Here's how the part is built. I have some questions about the finished solid (model axes, mm). Coordinates: 2 decimals unless noted, no trailing zeros. Write each loop counter-clockwise with the first axis right and the second up, starting at its lowest first coordinate (ties: lowest second). Pieces come first, ordered by that corner, then holes. Notation, with made-up numbers: M 33.5,6 L 59.5,6 A24 ccw 59.5,32 Z; hole C 35,24 d2. An arc over 180 degrees is marked long. Use one line per item in the form item = value. Start each with the question number.
1. I want a section at A-A, the plane y = -3.5. List the corners of the cut face in (x, z) for me.
2. I want a section at B-B, the plane y = 3. List the corners of the cut face in (x, z) for me, plus the area to 3 significant figures.
3. Please list where these lines run through material, in increasing order: line 1 along X through (y, z) = (2, 3.75); line 2 along X through (y, z) = (-1.75, 0.9); line 3 along Y through (x, z) = (0.75, 0.8). Write a range as [from, to].
4. Thinking about a two-plate mould opening in X: for faces 1 (the face through (2, -2, 0)), 2 (the face through (-0.6, 4.415, 1.972)), which applies, released by +X, released by -X, zero draft, split by the parting line, or undercut?
5. I'm going to push flat-ended pins straight in: pin 1 Ø2 at (x, z) = (1.5, 3) entering from +Y; pin 2 Ø1 at (y, z) = (-3.5, 1.5) entering from -X. Where does each tip first touch, or does it pass through?
from build123d import *

# Parameters (mm, degrees)
F0_R     = 4.49904
F1_DEPTH = 4


with BuildPart() as f1:
    # F0 (on Top) → F1 (new body)
    with BuildSketch(Plane.XY):
        with Locations((-0.014088, -0.045997)):
            Circle(F0_R)
        with BuildLine():
            ThreePointArc((1.873632, 0.614697), (1.909564, 0.501329), (1.938694, 0.386026))
            Line((1.938694, 0.386026), (2.203247, 0.410541))
            ThreePointArc((2.203247, 0.410541), (2.386026, 0.353941), (2.475248, 0.184674))
            ThreePointArc((2.475248, 0.184674), (2.418648, 0.001895), (2.249381, -0.087326))
            Line((2.249381, -0.087326), (1.984828, -0.111841))
            ThreePointArc((1.984828, -0.111841), (1.977381, -0.230533), (1.962892, -0.348573))
            Line((1.962892, -0.348573), (2.218436, -0.421282))
            ThreePointArc((2.218436, -0.421282), (2.368426, -0.540087), (2.390476, -0.730154))
            ThreePointArc((2.390476, -0.730154), (2.271671, -0.880144), (2.081604, -0.902195))
            Line((2.081604, -0.902195), (1.82606, -0.829486))
            ThreePointArc((1.82606, -0.829486), (1.776239, -0.937473), (1.720087, -1.042308))
            Line((1.720087, -1.042308), (1.93211, -1.20242))
            ThreePointArc((1.93211, -1.20242), (2.028581, -1.36415), (1.984828, -1.547313))
            ThreePointArc((1.984828, -1.547313), (1.819226, -1.649054), (1.630792, -1.601429))
            Line((1.630792, -1.601429), (1.41877, -1.441317))
            ThreePointArc((1.41877, -1.441317), (1.333304, -1.524015), (1.243073, -1.601486))
            Line((1.243073, -1.601486), (1.382939, -1.827377))
            ThreePointArc((1.382939, -1.827377), (1.413744, -2.016223), (1.301993, -2.17154))
            ThreePointArc((1.301993, -2.17154), (1.113147, -2.202345), (0.95783, -2.090593))
            Line((0.95783, -2.090593), (0.817964, -1.864702))
            ThreePointArc((0.817964, -1.864702), (0.708396, -1.910941), (0.596272, -1.950586))
            Line((0.596272, -1.950586), (0.645092, -2.211749))
            ThreePointArc((0.645092, -2.211749), (0.605598, -2.39897), (0.445286, -2.503429))
            ThreePointArc((0.445286, -2.503429), (0.258065, -2.463936), (0.153605, -2.303624))
            Line((0.153605, -2.303624), (0.104786, -2.042461))
            ThreePointArc((0.104786, -2.042461), (-0.014088, -2.045997), (-0.132961, -2.042461))
            Line((-0.132961, -2.042461), (-0.181781, -2.303624))
            ThreePointArc((-0.181781, -2.303624), (-0.28624, -2.463936), (-0.473461, -2.503429))
            ThreePointArc((-0.473461, -2.503429), (-0.633773, -2.39897), (-0.673267, -2.211749))
            Line((-0.673267, -2.211749), (-0.624448, -1.950586))
            ThreePointArc((-0.624448, -1.950586), (-0.736571, -1.910941), (-0.84614, -1.864702))
            Line((-0.84614, -1.864702), (-0.986006, -2.090593))
            ThreePointArc((-0.986006, -2.090593), (-1.141322, -2.202345), (-1.330168, -2.17154))
            ThreePointArc((-1.330168, -2.17154), (-1.44192, -2.016223), (-1.411114, -1.827377))
            Line((-1.411114, -1.827377), (-1.271248, -1.601486))
            ThreePointArc((-1.271248, -1.601486), (-1.361479, -1.524015), (-1.446945, -1.441317))
            Line((-1.446945, -1.441317), (-1.658968, -1.601429))
            ThreePointArc((-1.658968, -1.601429), (-1.847401, -1.649054), (-2.013004, -1.547313))
            ThreePointArc((-2.013004, -1.547313), (-2.056756, -1.36415), (-1.960285, -1.20242))
            Line((-1.960285, -1.20242), (-1.748263, -1.042308))
            ThreePointArc((-1.748263, -1.042308), (-1.804414, -0.937473), (-1.854236, -0.829486))
            Line((-1.854236, -0.829486), (-2.10978, -0.902195))
            ThreePointArc((-2.10978, -0.902195), (-2.299846, -0.880144), (-2.418652, -0.730154))
            ThreePointArc((-2.418652, -0.730154), (-2.396601, -0.540087), (-2.246611, -0.421282))
            Line((-2.246611, -0.421282), (-1.991067, -0.348573))
            ThreePointArc((-1.991067, -0.348573), (-2.005556, -0.230533), (-2.013004, -0.111841))
            Line((-2.013004, -0.111841), (-2.277557, -0.087326))
            ThreePointArc((-2.277557, -0.087326), (-2.446823, 0.001895), (-2.503423, 0.184674))
            ThreePointArc((-2.503423, 0.184674), (-2.414201, 0.353941), (-2.231422, 0.410541))
            Line((-2.231422, 0.410541), (-1.966869, 0.386026))
            ThreePointArc((-1.966869, 0.386026), (-1.937739, 0.501329), (-1.901807, 0.614697))
            Line((-1.901807, 0.614697), (-2.13964, 0.733124))
            ThreePointArc((-2.13964, 0.733124), (-2.263982, 0.878126), (-2.246611, 1.068349))
            ThreePointArc((-2.246611, 1.068349), (-2.105122, 1.193314), (-1.91677, 1.180705))
            Line((-1.91677, 1.180705), (-1.678938, 1.062279))
            ThreePointArc((-1.678938, 1.062279), (-1.610122, 1.159273), (-1.535663, 1.252005))
            Line((-1.535663, 1.252005), (-1.714655, 1.448349))
            ThreePointArc((-1.714655, 1.448349), (-1.779903, 1.616773), (-1.714655, 1.785197))
            ThreePointArc((-1.714655, 1.785197), (-1.529903, 1.866773), (-1.345151, 1.785197))
            Line((-1.345151, 1.785197), (-1.166159, 1.588853))
            ThreePointArc((-1.166159, 1.588853), (-1.066952, 1.654438), (-0.964022, 1.71401))
            Line((-0.964022, 1.71401), (-1.059999, 1.961755))
            ThreePointArc((-1.059999, 1.961755), (-1.05558, 2.153046), (-0.917192, 2.285184))
            ThreePointArc((-0.917192, 2.285184), (-0.725901, 2.280764), (-0.593763, 2.142376))
            Line((-0.593763, 2.142376), (-0.497786, 1.894631))
            ThreePointArc((-0.497786, 1.894631), (-0.381587, 1.919949), (-0.264088, 1.938317))
            Line((-0.264088, 1.938317), (-0.264088, 2.204003))
            ThreePointArc((-0.264088, 2.204003), (-0.190864, 2.38078), (-0.014088, 2.454003))
            ThreePointArc((-0.014088, 2.454003), (0.162689, 2.38078), (0.235912, 2.204003))
            Line((0.235912, 2.204003), (0.235912, 1.938317))
            ThreePointArc((0.235912, 1.938317), (0.353411, 1.919949), (0.469611, 1.894631))
            Line((0.469611, 1.894631), (0.565588, 2.142376))
            ThreePointArc((0.565588, 2.142376), (0.697726, 2.280764), (0.889016, 2.285184))
            ThreePointArc((0.889016, 2.285184), (1.027405, 2.153046), (1.031824, 1.961755))
            Line((1.031824, 1.961755), (0.935847, 1.71401))
            ThreePointArc((0.935847, 1.71401), (1.038777, 1.654438), (1.137983, 1.588853))
            Line((1.137983, 1.588853), (1.316975, 1.785197))
            ThreePointArc((1.316975, 1.785197), (1.501728, 1.866773), (1.68648, 1.785197))
            ThreePointArc((1.68648, 1.785197), (1.751728, 1.616773), (1.68648, 1.448349))
            Line((1.68648, 1.448349), (1.507488, 1.252005))
            ThreePointArc((1.507488, 1.252005), (1.581947, 1.159273), (1.650762, 1.062279))
            Line((1.650762, 1.062279), (1.888595, 1.180705))
            ThreePointArc((1.888595, 1.180705), (2.076947, 1.193314), (2.218436, 1.068349))
            ThreePointArc((2.218436, 1.068349), (2.235807, 0.878126), (2.111464, 0.733124))
            Line((2.111464, 0.733124), (1.873632, 0.614697))
        make_face(mode=Mode.SUBTRACT)
    extrude(amount=F1_DEPTH)


solid = f1.part
Answer list:
q1.outline = M -2.9,0 L 2.87,0 L 2.87,4 L -2.9,4 Z
q2.outline = M -3.33,0 L 3.3,0 L 3.3,4 L -3.33,4 Z
q2.area = 26.5 mm²
q3.line_1 = [-4.02, -1.07], [-0.54, -0.26], [0.24, 0.51], [1.04, 3.99]
q3.line_2 = [-4.18, -1.36], [1.34, 4.15]
q3.line_3 = [-4.48, -1.89], [2.3, 4.39]
q4.face_1 = zero draft
q4.face_2 = split by the parting line
q5.pin_1 = 4.42
q5.pin_2 = -3.41
